Part model, mm, in its own coordinate system. Round coordinates to 2 decimals unless told otherwise and drop trailing zeros. Loops run counter-clockwise (first coordinate to the right, second up) from the corner with the lowest first, then second, coordinate; pieces in that order, holes last. Notation, with made-up numbers: (59, 76.5) - (79, 76.5) arc R21 ccw to (79, 114.5) - close; hole circle Ø4 at (71, -10). An arc over 180 degrees is marked (long way). Write each question's results on one line, items separated by ' | '. Start each with the question number.
(1) Mould opens along X. For faces 1 (the face through (-20.874, 196.352, -0.919)), 2 (the face through (6.19, 97.39, 19.67)) say: released by +X, released by -X, zero draft, split by the parting line, or undercut.
(2) Flat gauge pins, fed straight in: P1, Ø10, axis at y = 145, z = 15.5, coming from the +X side; P2, Ø5, axis at x = 7, y = 47, coming from the +Z side; P3, Ø3, axis at x = -13.5, z = 19, coming from the +Y side. Where does each tip first touch, or does it go through?
(3) Cut at B-B, the plane x = 0. List the corners of the cut face in (y, z), then the cut area to 3 significant figures.
(4) Cut at A-A, the plane z = 0. List the corners of the cut face in (x, y), then the cut area to 3 significant figures.
(5) Drill centre lines: L1, parallel to X at y = 118, z = 0; L2, parallel to Z at x = 12, y = 79; L3, parallel to Z at x = 7.5, y = 161. Where is each one in solid material? Low to high.
(6) Cut at C-C, the plane y = 75. List the corners of the cut face in (x, z).
from build123d import *

# Parameters (mm, degrees)
SKETCH1_R           = 25
BOSS_EXTRUDE1_DEPTH = 198.941748
SKETCH2_R           = 20.620747434
CUT_EXTRUDE1_DEPTH  = 203.05894956


with BuildPart() as part:
    # Sketch1 → Boss-Extrude1 (new body)
    with BuildSketch(Plane(origin=(0, 0, 0), x_dir=(1, 0, 0), z_dir=(0, 1, 0))):
        with Locations(Location((0, 0, 0), (0, 0, 270))):
            Circle(SKETCH1_R)
    extrude(amount=BOSS_EXTRUDE1_DEPTH)

    # Sketch2 → Cut-Extrude1 (cut, through all)
    with BuildSketch(Plane(origin=(0, 0, 0), x_dir=(1, 0, 0), z_dir=(0, 1, 0))):
        with Locations(Location((0, 0, 0), (0, 0, 270))):
            Circle(SKETCH2_R)
    extrude(amount=CUT_EXTRUDE1_DEPTH, mode=Mode.SUBTRACT)

    # Chamfer1: read off the stored shape, not the designer's step
    # Chamfer1 outline → Chamfer1 (revolve, cut)
    with BuildSketch(Plane.XY):
        Polygon((25, 193.982213725), (25, 198.94174834), (20.620747434, 198.94174834), (20.620747434, 196.510576373), align=None)
        Polygon((25, 8.590165934), (20.620747434, 1.005077991), (20.620747434, 0), (25, 0), align=None)
    revolve(axis=Axis((0, 0, 0), (0, 1, 0)), mode=Mode.SUBTRACT)


solid = part.part
A:
1) face 1: split by the parting line | face 2: undercut
2) P1: x = 22.69 | P2: z = 24.59 | P3: y = 195.83
3) outline: (1.01, -20.62) - (8.59, -25) - (193.98, -25) - (196.51, -20.62) - close; (1.01, 20.62) - (196.51, 20.62) - (193.98, 25) - (8.59, 25) - close | area: 1,670 mm2
4) outline: (-25, 8.59) - (-20.62, 1.01) - (-20.62, 196.51) - (-25, 193.98) - close; (20.62, 1.01) - (25, 8.59) - (25, 193.98) - (20.62, 196.51) - close | area: 1,670 mm2
5) L1: -25 to -20.62, 20.62 to 25 | L2: -21.93 to -16.77, 16.77 to 21.93 | L3: -23.85 to -19.21, 19.21 to 23.85
6) outline: circle Ø50 at (0, 0); hole circle Ø41.24 at (0, 0)
